Verification items for this drawing (mm, ordinates from the low corner). A direction names the side the tool comes from. Round coordinates to 2 decimals unless told otherwise and drop trailing zeros. Loops run counter-clockwise (first coordinate to the right, second up) from the corner with the lowest first, then second, coordinate; pieces in that order, holes last. Notation, with made-up numbers: (89, 64) - (121, 64) arc R26 cw to (121, 100) - close; hole circle Ø3 at (27, 3). An arc over 180 degrees is marked (long way). Answer in a Markdown table with one row per item. Add a question column.
(1) Cross-section at A-A on x = 19.05. Count the separate pieces of the cut face and the enclosed holes in it, then the cut area to 3 significant figures.
(2) Cross-section at C-C on y = 6.35. Enter the section's corners in (x, z).
(3) Access from +Z, -Z, +X, -X, +Y, -Y to the whole of each face (thin tool, end or side, straight path). Record for the marked faces 1 and 2.
(4) Gauge pin test, flat ends, axial feed: pin 1 (3 mm diameter, centred on x = 9.445, z = 4.445, fed in from +Y); pin 2 (1.7 mm diameter, centred on x = 19.05, z = 4.445, fed in from -Y); pin 3 (9.5 mm diameter, centred on x = 10, y = 5.5, fed in from -Z); pin 4 (12 mm diameter, centred on x = 12.5, y = 3, fed in from +Z). Record the tip position at first contact, or that the pin passes through.
(5) Cross-section at B-B on z = 6.35. Enter the section's corners in (x, y), then the cut area to 3 significant figures.
(6) Thickness scan on line 1 along Z through (x, y) = (19.05, 21.3) (1 decimal); line 2 along Z through (x, y) = (3.15, 6.35); line 3 along X through (y, z) = (2.5, 2). Record the ranges inside material, lowest first.
(7) Mould release check, pull along Y, two halves, no side actions. Record for the marked faces 3, 4 and 5: +Y half, -Y half, draft (parallel to the pull), parting line (faces both ways), or undercut.
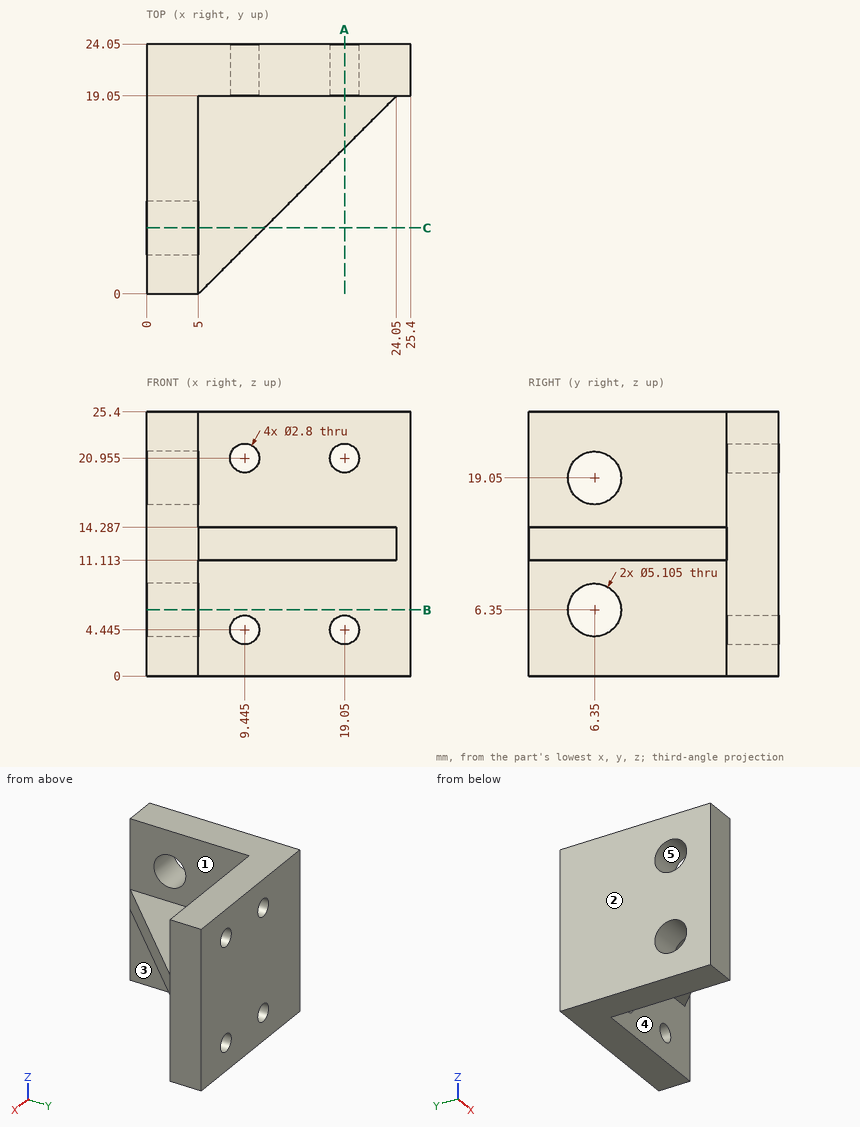
Answers:
| question | item | result |
|---|---|---|
| 1 | separate pieces | 3 |
| 1 | enclosed holes | 0 |
| 1 | area | 115 mm^2 |
| 2 | outline | (0, 0) - (5, 0) - (5, 3.8) - (0, 3.8) - close; (0, 8.9) - (5, 8.9) - (5, 11.11) - (11.35, 11.11) - (11.35, 14.29) - (5, 14.29) - (5, 16.5) - (0, 16.5) - close; (0, 21.6) - (5, 21.6) - (5, 25.4) - (0, 25.4) - close |
| 3 | face 1 | +Z, +X, -Y |
| 3 | face 2 | +Z, -Z, -X, +Y, -Y |
| 4 | pin 1 | stops at y = 24.05 |
| 4 | pin 2 | passes through |
| 4 | pin 3 | stops at z = 11.11 |
| 4 | pin 4 | stops at z = 14.29 |
| 5 | outline | (0, 0) - (5, 0) - (5, 3.8) - (0, 3.8) - close; (0, 8.9) - (5, 8.9) - (5, 19.05) - (25.4, 19.05) - (25.4, 24.05) - (0, 24.05) - close |
| 5 | area | 197 mm^2 |
| 6 | line 1 | z = 0 to 3, 5.8 to 19.6, 22.4 to 25.4 |
| 6 | line 2 | z = 0 to 3.8, 8.9 to 16.5, 21.6 to 25.4 |
| 6 | line 3 | x = 0 to 5 |
| 7 | face 3 | draft |
| 7 | face 4 | -Y half |
| 7 | face 5 | undercut |
